The listing builds one solid part. Answer for the finished solid, in the listing's coordinates (mm). A direction names the side the tool comes from. Coordinates: 2 decimals unless noted, no trailing zeros. Order: outer loops, then holes, each group sorted by start corner. A loop starts at its lowest first (then second) coordinate and runs counter-clockwise, first axis right, second up. Notation, with made-up numbers: (-10, 21) - (42, 21) arc R7 cw to (42, 31) - close; hole circle Ø4 at (47.5, 33). An arc over 180 degrees is marked (long way). Use a Markdown table: item, result. Add a question column.
Item 1: Find the intervals of material crossed by line 1 along Y through (x, z) = (114, -15); line 2 along Y through (x, z) = (114, -0.25); line 3 along X through (y, z) = (0.75, -6.75), in increasing order.
Item 2: For faces 4 (the flat face through (8.5, -9, -3)), 5 (the cylindrical face through (110, 0, 11)), 6 (the cylindrical face through (4.19, 9.667, 1.269)), 7 (the cylindrical face through (109.58, 4.06, -12.83)), determine the directions among +Z, -Z, +X, -X, +Y, -Y from which every point of the face is accessible in a straight line to the end or side of a thin tool.
Item 3: Flat-ended cylindrical pins translate along their axes: P1, Ø8, axis at x = 57.5, z = 0, coming from the -Y side; P2, Ø3, axis at x = 81.5, y = 6, coming from the -Z side; P3, Ø2.5, axis at x = 112.5, y = 0, coming from the -Z side; P4, Ø4, axis at x = 95, z = -9, coming from the +Y side. Find the tip coordinate at first contact, or state that the pin passes through.
Item 4: The part is cut by section B-B, the plane x = 114. Give the vertices of the cut face in (y, z).
Item 5: The mould has two halves that part along Y. Classify faces 1 (the cylindrical face through (55, 0, 6)), 2 (the flat face through (102, 8.2, 0)), 3 (the flat face through (114, -2, -12)): released by +Y, released by -Y, zero draft, split by the parting line, or undercut.
Item 6: The part is cut by section A-A, the plane z = 0. Give the vertices of the cut face in (x, y).
Item 7: The part is cut by section C-C, the plane x = 21.5. Give the vertices of the cut face in (y, z), then the cut area to 3 significant figures.
from build123d import *

# Parameters (mm, degrees)
SKETCH2_R                = 9.75
BOSS_EXTRUDE1_DEPTH      = 8.5
SKETCH3_R                = 6
BOSS_EXTRUDE2_DEPTH      = 93.5
FILLET1_R                = 3
SKETCH4_R                = 10
BOSS_EXTRUDE3_DEPTH      = 21
FILLET2_R                = 2
SKETCH5_R                = 6
BOSS_EXTRUDE4_DEPTH      = 13
BOSS_EXTRUDE4_DEPTH_BACK = 16
SKETCH6_R                = 4
CUT_EXTRUDE1_DEPTH       = 4
CUT_EXTRUDE2_REACH       = 27
SKETCH7_R                = 1.5
SKETCH8_R                = 4
CUT_EXTRUDE3_DEPTH       = 4


with BuildPart() as part:
    # Sketch2 → Boss-Extrude1 (new body)
    with BuildSketch(Plane(origin=(0, 0, 0), x_dir=(0, 0, -1), z_dir=(1, 0, 0))):
        Circle(SKETCH2_R)
    extrude(amount=BOSS_EXTRUDE1_DEPTH)

    # Sketch3 → Boss-Extrude2 (add)
    with BuildSketch(Plane(origin=(8.5, 0, 0), x_dir=(0, 0, -1), z_dir=(1, 0, 0))):
        Circle(SKETCH3_R)
    extrude(amount=BOSS_EXTRUDE2_DEPTH)

    # Fillet1
    fillet1_edges = [part.edges().sort_by_distance(p)[0] for p in [
        (8.5, 0, 6),
    ]]
    fillet(fillet1_edges, radius=FILLET1_R)

    # Sketch4 → Boss-Extrude3 (add)
    with BuildSketch(Plane(origin=(102, 0, 0), x_dir=(0, 0, -1), z_dir=(1, 0, 0))):
        Circle(SKETCH4_R)
    extrude(amount=BOSS_EXTRUDE3_DEPTH)

    # Fillet2
    fillet2_edges = [part.edges().sort_by_distance(p)[0] for p in [
        (102, 0, 6),
    ]]
    fillet(fillet2_edges, radius=FILLET2_R)

    # Sketch5 → Boss-Extrude4 (add, two sides)
    with BuildSketch(Plane.XY) as boss_extrude4_sk:
        with Locations((114, 0)):
            Circle(SKETCH5_R)
    extrude(amount=BOSS_EXTRUDE4_DEPTH)
    extrude(boss_extrude4_sk.sketch, amount=-BOSS_EXTRUDE4_DEPTH_BACK)

    # Sketch6 → Cut-Extrude1 (cut)
    with BuildSketch(Plane.XY.offset(13)):
        with Locations((114, 0)):
            Circle(SKETCH6_R)
    extrude(amount=-CUT_EXTRUDE1_DEPTH, mode=Mode.SUBTRACT)

    # Sketch7 → Cut-Extrude2 (cut, up to next)
    with BuildSketch(Plane.XY.offset(9), mode=Mode.PRIVATE) as cut_extrude2_sk1:
        with Locations((114, 0)):
            Circle(SKETCH7_R)
    cut_extrude2_tool1 = extrude(cut_extrude2_sk1.sketch, amount=-CUT_EXTRUDE2_REACH, mode=Mode.PRIVATE) & part.part
    add(cut_extrude2_tool1.solids().sort_by_distance((114, 0, 9))[0], mode=Mode.SUBTRACT)

    # Sketch8 → Cut-Extrude3 (cut)
    with BuildSketch(Plane(origin=(0, 0, -16), x_dir=(-1, 0, 0), z_dir=(0, 0, -1))):
        with Locations((-114, 0)):
            Circle(SKETCH8_R)
    extrude(amount=-CUT_EXTRUDE3_DEPTH, mode=Mode.SUBTRACT)


solid = part.part
Solution:
| question | item | result |
|---|---|---|
| 1 | line 1 | y = -6 to -4, 4 to 6 |
| 1 | line 2 | y = -10 to -1.5, 1.5 to 10 |
| 1 | line 3 | x = 0 to 9.47, 101.59 to 112.7, 115.3 to 123 |
| 2 | face 4 | none |
| 2 | face 5 | +Z |
| 2 | face 6 | -X |
| 2 | face 7 | -Z |
| 3 | P1 | stops at y = -6 |
| 3 | P2 | stops at z = -3.97 |
| 3 | P3 | stops at z = -12 |
| 3 | P4 | passes through |
| 4 | outline | (-6, -16) - (-4, -16) - (-4, -12) - (-1.5, -12) - (-1.5, 9) - (-4, 9) - (-4, 13) - (-6, 13) - (-6, 8) arc R10 ccw to (-6, -8) - close; (1.5, -12) - (4, -12) - (4, -16) - (6, -16) - (6, -8) arc R10 ccw to (6, 8) - (6, 13) - (4, 13) - (4, 9) - (1.5, 9) - close |
| 5 | face 1 | split by the parting line |
| 5 | face 2 | zero draft |
| 5 | face 3 | undercut |
| 6 | outline | (0, -9.75) - (8.5, -9.75) - (8.5, -9) arc R3 cw to (11.5, -6) - (100, -6) arc R2 cw to (102, -8) - (102, -10) - (123, -10) - (123, 10) - (102, 10) - (102, 8) arc R2 cw to (100, 6) - (11.5, 6) arc R3 cw to (8.5, 9) - (8.5, 9.75) - (0, 9.75) - close; hole circle Ø3 at (114, 0) |
| 7 | outline | circle Ø12 at (0, 0) |
| 7 | area | 113 mm2 |
